CAD build for the part. Positions are in the model's coordinates, mm. Face numbers are marked on the shaded views. A direction names the side the tool comes from. Round coordinates to 2 decimals unless told otherwise and drop trailing zeros. Loops run counter-clockwise (first coordinate to the right, second up) from the corner with the lowest first, then second, coordinate; pieces in that order, holes last.
```python
from build123d import *

# Parameters (mm, degrees)
ESQUISSE1_R        = 4.8895
ESQUISSE1_R_2      = 2.032
BOSS_EXTRU_1_DEPTH = 13.335


with BuildPart() as part:
    # Esquisse1 → Boss.-Extru.1 (new, symmetric)
    with BuildSketch(Plane.XY):
        Circle(ESQUISSE1_R)
        Circle(ESQUISSE1_R_2, mode=Mode.SUBTRACT)
    extrude(amount=BOSS_EXTRU_1_DEPTH, both=True)

    # Esquisse2 → Révolution1 (revolve)
    with BuildSketch(Plane(origin=(0, 0, 0), x_dir=(0, 0, -1), z_dir=(1, 0, 0)), mode=Mode.PRIVATE) as r_volution1_sk:
        Polygon((-0.635, 4.8895), (-13.335, 8.0645), (-13.335, 4.8895), align=None)
    r_volution1 = revolve(r_volution1_sk.sketch.rotate(Axis((0, 0, 0), (0, 0, 1)), 90), axis=Axis((0, 0, 0), (0, 0, 1)))

    # Symétrie1: Révolution1 across plane
    add(r_volution1.mirror(Plane.XY))


solid = part.part
```
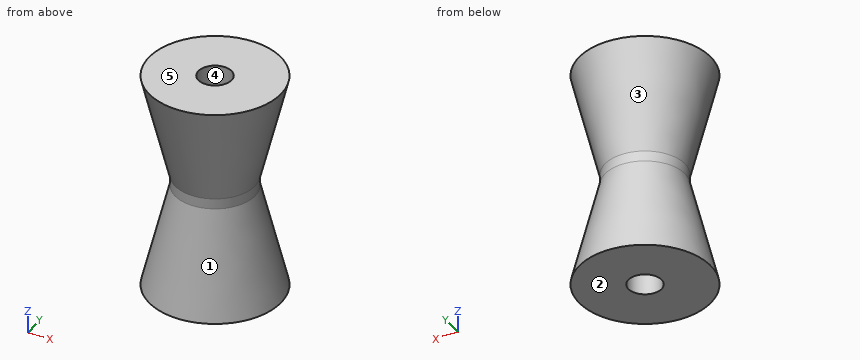
Item 1: Probe line 1 (Y direction, x = 0.75, z = -7.5); line 2 (Y direction, x = 0, z = 1.75); line 3 (X direction, y = 1.25, z = -9.5). List the from-to ranges inside material, lowest first.
Answers follow:
line 1: y = -6.56 to -1.89, 1.89 to 6.56
line 2: y = -5.17 to -2.03, 2.03 to 5.17
line 3: x = -6.99 to -1.6, 1.6 to 6.99
Item 2: Cut at D-D, the plane z = -9. Give the cut face in (x, y).
Answers follow:
outline: circle Ø13.96 at (0, 0); hole circle Ø4.06 at (0, 0)
Item 3: 3-axis set-ups, long thin cutter, end or side, ignore diameter. For the marked faces 1 and 2: which of +Z, -Z, +X, -X, +Y, -Y reach the whole face in a straight line?
Answers follow:
face 1: none
face 2: -Z, +X, -X, +Y, -Y
Item 4: Cut at C-C, the plane z = 7.25. Give the cut face in (x, y).
Answers follow:
outline: circle Ø13.09 at (0, 0); hole circle Ø4.06 at (0, 0)
Item 5: Two-plate mould, pull along X, no slides. Class the marked faces 3, 4 and 5: released by +X, released by -X, zero draft, split by the parting line, or undercut.
Answers follow:
face 3: split by the parting line
face 4: undercut
face 5: zero draft
Item 6: Cut at A-A, the plane x = 0. Give the cut face in (y, z) (1 decimal), plus the area to 3 significant figures.
Answers follow:
outline: (-8.1, -13.3) - (-2, -13.3) - (-2, 13.3) - (-8.1, 13.3) - (-4.9, 0.6) - (-4.9, -0.6) - close; (2, -13.3) - (8.1, -13.3) - (4.9, -0.6) - (4.9, 0.6) - (8.1, 13.3) - (2, 13.3) - close
area: 233 mm2
Item 7: Flat gauge pins, fed straight in: P1, Ø1.5, axis at x = 2, z = -5, coming from the -Y side; P2, Ø4, axis at x = 0.5, z = 9, coming from the +Y side; P3, Ø5, axis at x = 5, z = -7, coming from the +Y side. Where does each tip first touch, or does it go through?
Answers follow:
P1: stops at y = -5.93
P2: stops at y = 7.47
P3: stops at y = 6.17
